```python
from build123d import *

# Parameters (mm, degrees)
SKETCH1_W             = 3.207256709
SKETCH1_H             = 44
BOSS_EXTRUDE2_DEPTH   = 33
BOSS_EXTRUDE2_2_DEPTH = 33
BOSS_EXTRUDE3_DEPTH   = 40
CHAMFER4_SIZE         = 4.23
SKETCH2_W             = 8
SKETCH2_H             = 10
BOSS_EXTRUDE4_DEPTH   = 1.2
SKETCH3_W             = 10
SKETCH3_H             = 10
BOSS_EXTRUDE5_DEPTH   = 1.2
SKETCH4_W             = 3.207256709
SKETCH4_H             = 10
CUT_EXTRUDE1_DEPTH    = 15


with BuildPart() as part:
    # Sketch1 → Boss-Extrude2 (new body)
    with BuildSketch(Plane(origin=(0, 0, 0), x_dir=(1, 0, 0), z_dir=(0, 1, 0))):
        with Locations((-22.853628355, 0)):
            Rectangle(SKETCH1_W, SKETCH1_H)
    extrude(amount=BOSS_EXTRUDE2_DEPTH)



with BuildPart() as body_2:
    # Sketch1 → Boss-Extrude2 2 (new body)
    with BuildSketch(Plane(origin=(0, 0, 0), x_dir=(1, 0, 0), z_dir=(0, 1, 0))):
        Polygon((23.75, 22), (21.25, 22), (21.25, -22), (24.457256709, -22), (24.457256709, 22), align=None)
    extrude(amount=BOSS_EXTRUDE2_2_DEPTH)


with BuildPart() as part_1:
    add(part.part)

    add(body_2.part)  # Boss-Extrude3 merges body 2
    # Sketch1_6 → Boss-Extrude3 (add)
    with BuildSketch(Plane(origin=(0, 0, 0), x_dir=(1, 0, 0), z_dir=(0, 1, 0))):
        Polygon((-26.85, 28.85), (-25.85, 28.85), (-25.85, 25.85), (25.85, 25.85), (25.85, 28.85), (26.85, 28.85), (26.85, 30.6), (25.85, 30.6), (25.85, 32.5), (29.6, 32.5), (29.6, 22), (-29.6, 22), (-29.6, 32.5), (-25.85, 32.5), (-25.85, 30.6), (-26.85, 30.6), align=None)
    extrude(amount=BOSS_EXTRUDE3_DEPTH)

    # Chamfer4
    chamfer4_edges = [part_1.edges().sort_by_distance(p)[0] for p in [
        (21.25, 16.5, -22),
        (-21.25, 16.5, -22),
    ]]
    chamfer(chamfer4_edges, length=CHAMFER4_SIZE)

    # Sketch2 → Boss-Extrude4 (add)
    with BuildSketch(Plane(origin=(-19.51, 0, -19.51), x_dir=(0.7071067811865509, 0, -0.7071067811865442), z_dir=(0.7071067811865442, 0, 0.7071067811865509))):
        with Locations((0.603606398, 16.5)):
            Rectangle(SKETCH2_W, SKETCH2_H)
    extrude(amount=BOSS_EXTRUDE4_DEPTH)

    # Sketch3 → Boss-Extrude5 (add)
    with BuildSketch(Plane(origin=(19.51, 0, -19.51), x_dir=(0.7071067811865442, 0, 0.7071067811865509), z_dir=(-0.7071067811865509, 0, 0.7071067811865442))):
        with Locations((-0.530330086, 16.5)):
            Rectangle(SKETCH3_W, SKETCH3_H)
    extrude(amount=BOSS_EXTRUDE5_DEPTH)

    # Sketch4 → Cut-Extrude1 (cut)
    with BuildSketch(Plane(origin=(0, 33, 0), x_dir=(1, 0, 0), z_dir=(0, 1, 0))):
        with Locations((-22.853628355, 0)):
            Rectangle(SKETCH4_W, SKETCH4_H)
    extrude(amount=-CUT_EXTRUDE1_DEPTH, mode=Mode.SUBTRACT)


solid = part_1.part
```
The listing builds one solid part. Answer for the finished solid, in the listing's coordinates (mm). A direction names the side the tool comes from. Round coordinates to 2 decimals unless told otherwise and drop trailing zeros. Loops run counter-clockwise (first coordinate to the right, second up) from the corner with the lowest first, then second, coordinate; pieces in that order, holes last. Notation, with made-up numbers: (-34, 35.25) - (-14, 35.25) arc R6 cw to (-14, 45.25) - close; hole circle Ø3 at (-2.75, 85.25). An arc over 180 degrees is marked (long way). Use one line per item in the form item = value. Start each with the question number.
1. The part is cut by section D-D on y = 10. Determine the outline of the cut face in (x, z), then the cut area to 3 significant figures.
2. Given pin 1 Ø0.5 at (x, y) = (26.5, 12.5) entering from +Z; pin 2 Ø10 at (y, z) = (8.5, -3) entering from -X; pin 3 Ø3 at (x, z) = (-18.5, -18.5) entering from +Y, each flat-ended and moving along its own axis, determine where each tip first touches the part or whether it passes through.
3. The part is cut by section B-B on z = 15. Determine the outline of the cut face in (x, y).
4. For a pull along X with two mould halves and no side action, classify faces 5 (the face through (19.16, 27.17, -19.86)), 6 (the face through (0, 0, -24)), 7 (the face through (-24.457, 16, 0)) as pulls with the +X half, pulls with the -X half, needs draft (parallel to the pull), parting line crosses it, or undercut.
5. Consider line 1 (Z direction, x = -23.5, y = 21.5); line 2 (X direction, y = 20.5, z = -14); line 3 (Z direction, x = 23.5, y = 16.5). Determine where each line is inside the solid, lowest interval first. Write a range as [from, to].
6. A tool of negligible diameter and unlimited length cuts with its end or side. For faces 1 (the face through (25.85, 20, -27)), 2 (the face through (22, 33, 0)), 3 (the face through (-19.16, 27.17, -19.86)), 4 (the face through (18.245, 16.57, -19.078)), from which of +Z, -Z, +X, -X, +Y, -Y can it reach the whole face along a straight path? Write none if from no direction.
7. The part is cut by section C-C on x = -22.5. Determine the outline of the cut face in (y, z), then the cut area to 3 significant figures.
Geometry check:
q1.outline = (-29.6, -32.5) - (-25.85, -32.5) - (-25.85, -30.6) - (-26.85, -30.6) - (-26.85, -28.85) - (-25.85, -28.85) - (-25.85, -25.85) - (25.85, -25.85) - (25.85, -28.85) - (26.85, -28.85) - (26.85, -30.6) - (25.85, -30.6) - (25.85, -32.5) - (29.6, -32.5) - (29.6, -22) - (24.46, -22) - (24.46, 22) - (21.25, 22) - (21.25, -17.77) - (17.02, -22) - (-17.02, -22) - (-21.25, -17.77) - (-21.25, 22) - (-24.46, 22) - (-24.46, -22) - (-29.6, -22) - close
q1.area = 574 mm^2
q2.pin_1 = -22
q2.pin_2 = -24.46
q2.pin_3 = 33
q3.outline = (-24.46, 0) - (-21.25, 0) - (-21.25, 33) - (-24.46, 33) - close; (21.25, 0) - (24.46, 0) - (24.46, 33) - (21.25, 33) - close
q4.face_5 = undercut
q4.face_6 = needs draft
q4.face_7 = pulls with the -X half
q5.line_1 = [-25.85, -5], [5, 22]
q5.line_2 = [-24.46, -21.25], [21.25, 24.46]
q5.line_3 = [-25.85, 22]
q6.face_1 = -Z, +Y, -Y
q6.face_2 = +Z, +X, -X, +Y
q6.face_3 = +Z, +Y
q6.face_4 = +Z, +Y, -Y
q7.outline = (0, -25.85) - (40, -25.85) - (40, -22) - (33, -22) - (33, -5) - (18, -5) - (18, 5) - (33, 5) - (33, 22) - (0, 22) - close
q7.area = 1,460 mm^2
